The listing builds one solid part. Answer for the finished solid, in the listing's coordinates (mm). Give positions to 0.01 mm unless a question says otherwise; leave off trailing zeros. Write each loop counter-clockwise with the first axis right and the second up, starting at its lowest first coordinate (ties: lowest second). Pieces come first, ordered by that corner, then holes. Notation, with made-up numbers: (56, 63) - (62, 63) arc R32 ccw to (62, 92) - close; hole circle Ø10 at (66.25, -16). An arc over 180 degrees is marked (long way). Return JSON: item names as keys, results as strings.
from build123d import *

# Parameters (mm, degrees)
SKETCH1_R                      = 9.525
EXTRUDE1_DEPTH                 = 3.175
F_5_16_0_3125_DIAMETER_HOLE1_D = 7.9375


with BuildPart() as part:
    # Sketch1 → Extrude1 (new, symmetric)
    with BuildSketch(Plane.XY):
        Circle(SKETCH1_R)
    extrude(amount=EXTRUDE1_DEPTH, both=True)

    # 5/16 (0.3125) Diameter Hole1 (through all)
    with Locations(Plane.XY.offset(3.175)):
        with Locations((0, -1.5875)):
            Hole(F_5_16_0_3125_DIAMETER_HOLE1_D / 2)


solid = part.part
Item 1: A cutting plane is placed at B-B on y = 0. Determine the outline of the cut face in (x, z) (3 decimals).
Answer below:
{"outline": "(-9.525, -3.175) - (-3.637, -3.175) - (-3.637, 3.175) - (-9.525, 3.175) - close; (3.637, -3.175) - (9.525, -3.175) - (9.525, 3.175) - (3.637, 3.175) - close"}
Item 2: A cutting plane is placed at A-A on x = 0. Determine the outline of the cut face in (y, z) (3 decimals).
Answer below:
{"outline": "(-9.525, -3.175) - (-5.556, -3.175) - (-5.556, 3.175) - (-9.525, 3.175) - close; (2.381, -3.175) - (9.525, -3.175) - (9.525, 3.175) - (2.381, 3.175) - close"}
Item 3: Consider L1, parallel to Y at x = 0, z = -1.5 (3 decimals); L2, parallel to Y at x = 1, z = 0.75; L3, parallel to X at y = -3.75, z = 1. Determine where each line is inside the solid, lowest interval first.
Answer below:
{"L1": "y = -9.525 to -5.556, 2.381 to 9.525", "L2": "y = -9.47 to -5.43, 2.25 to 9.47", "L3": "x = -8.76 to -3.33, 3.33 to 8.76"}
Item 4: The mould has two halves that part along Y. Classify faces 1 (the face through (2, 2.3, 3.175)), 2 (the face through (-7.559, -5.796, 0.044)), 3 (the face through (0.86, -5.46, -0.04)): +Y half, -Y half, draft (parallel to the pull), parting line (faces both ways), or undercut.
Answer below:
{"face 1": "draft", "face 2": "parting line", "face 3": "undercut"}
Item 5: A cutting plane is placed at D-D on x = -7. Determine the outline of the cut face in (y, z) (3 decimals).
Answer below:
{"outline": "(-6.46, -3.175) - (6.46, -3.175) - (6.46, 3.175) - (-6.46, 3.175) - close"}
Item 6: A flat-ended cylindrical pin translates along its axis: P1, Ø7, axis at x = 0, y = -1.59, coming from the +Z side. Find the tip coordinate at first contact, or state that the pin passes through.
Answer below:
{"P1": "passes through"}
